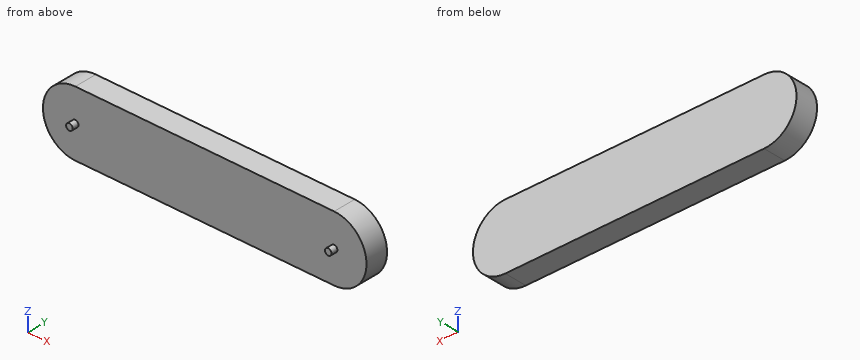
```python
from build123d import *

# Parameters (mm, degrees)
BOSS_EXTRUDE1_DEPTH = 70
SKETCH3_R           = 10
BOSS_EXTRUDE2_DEPTH = 20
SKETCH4_R           = 10
BOSS_EXTRUDE3_DEPTH = 20


with BuildPart() as part:
    # Sketch2 → Boss-Extrude1 (new body)
    with BuildSketch(Plane(origin=(0, 0, 0), x_dir=(1, 0, 0), z_dir=(0, 1, 0))):
        with BuildLine():
            Line((0, 100), (800, 100))
            ThreePointArc((800, 100), (900, 0), (800, -100))
            Line((800, -100), (0, -100))
            ThreePointArc((0, -100), (-100, 0), (0, 100))
        make_face()
    extrude(amount=BOSS_EXTRUDE1_DEPTH)

    # Sketch3 → Boss-Extrude2 (add)
    with BuildSketch(Plane.XZ):
        Circle(SKETCH3_R)
    extrude(amount=BOSS_EXTRUDE2_DEPTH)

    # Sketch4 → Boss-Extrude3 (add)
    with BuildSketch(Plane.XZ):
        with Locations((800, 0)):
            Circle(SKETCH4_R)
    extrude(amount=BOSS_EXTRUDE3_DEPTH)


solid = part.part
```
Input: part model. Units: mm. Frame: model coordinates. Give positions to 0.01 mm unless a question says otherwise; leave off trailing zeros. Order: outer loops, then holes, each group sorted by start corner. A loop starts at its lowest first (then second) coordinate and runs counter-clockwise, first axis right, second up.
1. Section C-C on y = 13.5. Return the cut outline in (x, z), and give its area (3 significant figures).
Derived:
outline: (0, -100) - (800, -100) arc R100 ccw to (800, 100) - (0, 100) arc R100 ccw to start
area: 191,000 mm2
2. Section B-B on x = 759. Return the cut outline in (y, z), and give its area (3 significant figures).
Derived:
outline: (0, -100) - (70, -100) - (70, 100) - (0, 100) - close
area: 14,000 mm2
3. Material intervals for L1, parallel to Y at x = 811.5, z = 58; L2, parallel to X at y = -10, z = 5; L3, parallel to X at y = 40.5, z = 16, sorted ascending.
Derived:
L1: y = 0 to 70
L2: x = -8.66 to 8.66, 791.34 to 808.66
L3: x = -98.71 to 898.71
4. Section A-A on z = 0. Return the cut outline in (x, y), and give its area (3 significant figures).
Derived:
outline: (-100, 0) - (-10, 0) - (-10, -20) - (10, -20) - (10, 0) - (790, 0) - (790, -20) - (810, -20) - (810, 0) - (900, 0) - (900, 70) - (-100, 70) - close
area: 70,800 mm2
5. Pin query (flat end, axial travel): pin 1 (8 mm diameter, centred on y = 1.5, z = -26, fed in from +X); pin 2 (8 mm diameter, centred on x = 595.5, z = 46, fed in from -Y); pin 3 (8 mm diameter, centred on y = 9, z = 67.5, fed in from +X). Return the tip coordinate at first contact, or that it passes through.
Derived:
pin 1: stops at x = 897.55
pin 2: stops at y = 0
pin 3: stops at x = 877.25
